For this review, take the finished solid that the model builds, in its own axes (mm). A direction names the side the tool comes from. Coordinates: 2 decimals unless noted, no trailing zeros. Order: outer loops, then holes, each group sorted by start corner. A loop starts at its lowest first (then second) coordinate and runs counter-clockwise, first axis right, second up. Notation, with made-up numbers: (77, -17) - (133, -17) arc R23 ccw to (133, 5) - close; hole circle Ø2 at (83, 75). An arc over 180 degrees is marked (long way). One line per item, written item: value. Start each with the question number.
(1) Consider section C-C on x = 21. Write out the cut boundary in (y, z).
(2) For faces 1 (the flat face through (0, 19, 520)), 2 (the flat face through (23, 4.762, 520)), list the 3-axis set-ups (+Z, -Z, +X, -X, +Y, -Y) from which the entire face can be reached by the end or side of a thin tool; tool diameter is ignored.
(3) To check wall thickness, follow line 1 along X through (y, z) = (24, 778); line 2 along Z through (x, y) = (18, 2.5). State the ranges of each line that lie inside material, in increasing order.
(4) Consider section A-A on z = 89. Write out the cut boundary in (x, y), then the cut area to 3 significant figures.
(5) Clearance check with flat-ended pins moving along their axes: pin 1 (1.5 mm diameter, centred on x = 10, z = 192, fed in from +Y); pin 2 (1.5 mm diameter, centred on x = 7, y = 16, fed in from -Z); pin 3 (6 mm diameter, centred on x = 8.5, z = 176.5, fed in from +Y); pin 4 (8 mm diameter, centred on y = 25.5, z = 470.5, fed in from +X). State where each tip first meets the part, or that it passes through.
(6) Consider section B-B on y = 20. Write out the cut boundary in (x, z).
Autodesk Inventor part; units mm, degrees
ref_plane "Start plane" through (0, 0, 0) normal (0, 0, 1) x (1, 0, 0)
ref_plane "End plane" through (0, 0, 1054.1) normal (0, 0, 1) x (1, 0, 0)
ref_plane "Work Plane4" through (19.05, 0, 1054.1) normal (0, 0.7071, 0.7071) x (1, 0, 0)
ref_plane "Start plane" through (0, 0, 0) normal (0, 0, 1) x (1, 0, 0)
ref_plane "End plane" through (0, 0, 1054.1) normal (0, 0, 1) x (1, 0, 0)
sketch "Sketch" plane through (0, 0, 0) normal (0, 0, 1) x (1, 0, 0)
  line L0 (38.1, 0) -> (0, 0)
  line L1 (0, 0) -> (0, 38.1)
  line L2 (0, 38.1) -> (2.4765, 38.1)
  line L3 (4.7625, 35.814) -> (4.7625, 9.5885)
  line L4 (9.5885, 4.7625) -> (35.814, 4.7625)
  line L5 (38.1, 2.4765) -> (38.1, 0)
  line L6 (0, -11.0414) -> (0, 31.5385) construction
  line L7 (-11.0414, 0) -> (31.5385, 0) construction
  arc A0 (4.7625, 9.5885) -> (9.5885, 4.7625) centre (9.5885, 9.5885) ccw
  arc A1 (4.7625, 35.814) -> (2.4765, 38.1) centre (2.4765, 35.814) ccw
  arc A2 (38.1, 2.4765) -> (35.814, 4.7625) centre (35.814, 2.4765) ccw
  line L8 (0, 48.4964) -> (0, -20.9644) construction
  line L9 (-20.9644, 0) -> (48.4964, 0) construction
  point P0 (4.7625, 38.1)
  point P1 (4.7625, 4.7625)
  point P2 (38.1, 4.7625)
  dimension "d0" = 38.1
  dimension "d1" = 38.1
  dimension "d2" = 4.7625
  dimension "d3" = 4.7625
  dimension "d10" = 0
  dimension "d11" = 0
  dimension "d14" = 4.826
  dimension "d15" = 2.286
extrude "Body" add sketch "Sketch" along normal up to surface (1054.1 mm away) from surface at 0
sketch "Sketch3" plane through (0, 0, 0) normal (0, 0, 1) x (1, 0, 0)
  line L0 (0, 0) -> (10, 0)
ref_plane "Work Plane3" through (0, 0, 0) normal (0, -1, 0) x (1, 0, 0)
sketch "Sketch4" plane through (0, 0, 0) normal (0, -1, 0) x (1, 0, 0)
  line L0 (-2, 0) -> (12, 0)
  line L1 (-2, 1054.1) -> (12, 1054.1)
  dimension "d17" = 1054.1
ref_plane "Work Plane4" through (19.05, 0, 1054.1) normal (0, 0.7071, 0.7071) x (1, 0, 0)
split "Split1" plane through (19.05, 0, 1054.1) removes the side toward (0, 0.7071, 0.7071)
ref_plane "Work Plane5" through (19.05, 0, 0) normal (0, 0.7071, -0.7071) x (1, 0, 0)
split "Split2" plane through (19.05, 0, 0) removes the side toward (0, 0.7071, -0.7071)
equation "\"d0\" = G_H"
equation "\"d1\" = G_H"
equation "\"d2\" = G_T"
equation "\"d3\" = G_T"
equation "\"d14\" = G_IR"
equation "\"d15\" = G_ER"
equation "\"d4\" = G_L"
equation "\"G_H\" = 38.1"
equation "\"G_T\" = 4.7625"
equation "\"G_ER\" = 2.286"
equation "\"G_IR\" = 4.826"
equation "\"G_L\" = d17"
equation "\"ex\" = 0"
equation "\"G_OFFSET_START\" = 0"
equation "\"G_OFFSET_END\" = 0"
equation "\"d13\" = G_OFFSET_END + B_L"
equation "\"B_L\" = 1054.1"
properties part number "AISC - L 1.5 x 1.5 x 3/16 - 41.5" material "Aluminum 6061-AHC"
Geometry check:
1. outline: (0, 0) - (4.76, 4.76) - (4.76, 1049.34) - (0, 1054.1) - close
2. face 1: +Z, -Z, -X, +Y, -Y
2. face 2: +Z, -Z, +X, +Y
3. line 1: x = 0 to 4.76
3. line 2: z = 2.5 to 1051.6
4. outline: (0, 0) - (38.1, 0) - (38.1, 2.48) arc R2.29 ccw to (35.81, 4.76) - (9.59, 4.76) arc R4.83 cw to (4.76, 9.59) - (4.76, 35.81) arc R2.29 ccw to (2.48, 38.1) - (0, 38.1) - close
4. area: 343 mm^2
5. pin 1: stops at y = 4.77
5. pin 2: passes through
5. pin 3: stops at y = 7.02
5. pin 4: stops at x = 4.76
6. outline: (0, 20) - (4.76, 20) - (4.76, 1034.1) - (0, 1034.1) - close
